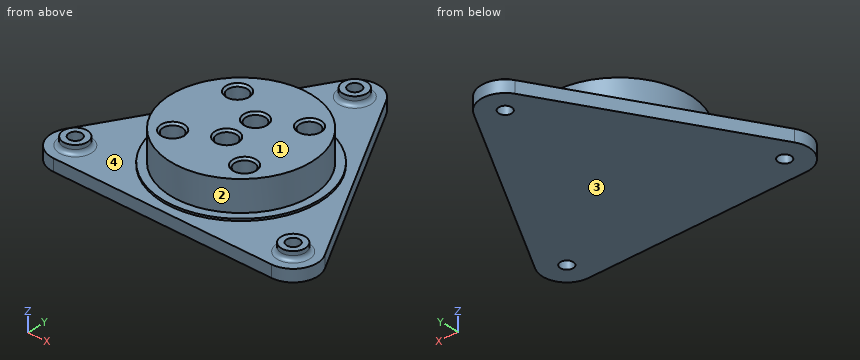
```python
from build123d import *

# Parameters (mm, degrees)
SKETCH2_R           = 1.6
CUT_EXTRUDE1_DEPTH  = 65.58327957
SKETCH3_R           = 2.4
CUT_EXTRUDE2_DEPTH  = 4
SKETCH5_OUTSIDE_W   = 117.55
SKETCH5_OUTSIDE_H   = 117.55
CUT_EXTRUDE4_DEPTH  = 65.140470843
CHAMFER1_SIZE       = 0.5
SKETCH6_R           = 3
SKETCH6_R_2         = 1.6
BOSS_EXTRUDE1_DEPTH = 2
FILLET1_R           = 1
SKETCH7_R           = 1.75
CUT_EXTRUDE5_DEPTH  = 6


with BuildPart() as part:
    # Sketch1 → Revolve1 (revolve)
    with BuildSketch(Plane(origin=(0, 0, 0), x_dir=(0, 0, -1), z_dir=(1, 0, 0)), mode=Mode.PRIVATE) as revolve1_sk:
        Polygon((0, 0), (0, 45), (-3, 45), (-3, 19.5), (-3.5, 19.5), (-3.5, 17.5), (-11, 17.5), (-11, 0), align=None)
    revolve(revolve1_sk.sketch.rotate(Axis((0, 0, 11), (0, 0, -1)), 90), axis=Axis((0, 0, 11), (0, 0, -1)))

    # Sketch2 → Cut-Extrude1 (cut, through all)
    with BuildSketch(Plane(origin=(0, 0, 0), x_dir=(-1, 0, 0), z_dir=(0, 0, -1))):
        with Locations(Location((0, 31.5, 0), (0, 0, 90))):
            Circle(SKETCH2_R)
        with Locations(Location((27.279800219, -15.75, 0), (0, 0, 90))):
            Circle(SKETCH2_R)
        with Locations(Location((-27.279800219, -15.75, 0), (0, 0, 90))):
            Circle(SKETCH2_R)
    extrude(amount=-CUT_EXTRUDE1_DEPTH, mode=Mode.SUBTRACT)

    # Sketch3 → Cut-Extrude2 (cut)
    with BuildSketch(Plane.XY.offset(11)):
        with Locations((0, 4)):
            Circle(SKETCH3_R)
        with Locations((0, -4)):
            Circle(SKETCH3_R)
        with Locations((-9, 9)):
            Circle(SKETCH3_R)
        with Locations((9, 9)):
            Circle(SKETCH3_R)
        with Locations((9, -9)):
            Circle(SKETCH3_R)
        with Locations((-9, -9)):
            Circle(SKETCH3_R)
    extrude(amount=-CUT_EXTRUDE2_DEPTH, mode=Mode.SUBTRACT)

    # Sketch5 outside → Cut-Extrude4 (cut, through all)
    with BuildSketch(Plane(origin=(0, 0, 3), x_dir=(-1, 0, 0), z_dir=(0, 0, -1))):
        Rectangle(SKETCH5_OUTSIDE_W, SKETCH5_OUTSIDE_H)
        with BuildLine():
            Line((-5.196152423, 34.5), (-32.475952642, -12.75))
            ThreePointArc((-32.475952642, -12.75), (-32.475952642, -18.75), (-27.279800219, -21.75))
            Line((-27.279800219, -21.75), (27.279800219, -21.75))
            ThreePointArc((27.279800219, -21.75), (32.475952642, -18.75), (32.475952642, -12.75))
            Line((32.475952642, -12.75), (5.196152423, 34.5))
            ThreePointArc((5.196152423, 34.5), (0, 37.5), (-5.196152423, 34.5))
        make_face(mode=Mode.SUBTRACT)
    extrude(amount=CUT_EXTRUDE4_DEPTH, mode=Mode.SUBTRACT)

    # Chamfer1
    chamfer1_edges = [part.edges().sort_by_distance(p)[0] for p in [
        (-2.4, -4, 11),
        (-11.4, 9, 11),
        (6.6, 9, 11),
        (6.6, -9, 11),
        (-11.4, -9, 11),
        (-2.4, 4, 11),
    ]]
    chamfer(chamfer1_edges, length=CHAMFER1_SIZE)

    # Sketch6 → Boss-Extrude1 (add)
    # profile 1 of 3: a face of its own
    with BuildSketch(Plane.XY.offset(3)):
        with Locations(Location((0, 31.5, 0), (0, 0, 180))):
            Circle(SKETCH6_R)
        with Locations(Location((0, 31.5, 0), (0, 0, 90))):
            Circle(SKETCH6_R_2, mode=Mode.SUBTRACT)
    # profile 2 of 3: a face of its own
    with BuildSketch(Plane.XY.offset(3)):
        with Locations(Location((-27.279800219, -15.75, 0), (0, 0, 180))):
            Circle(SKETCH6_R)
        with Locations(Location((-27.279800219, -15.75, 0), (0, 0, 90))):
            Circle(SKETCH6_R_2, mode=Mode.SUBTRACT)
    # profile 3 of 3: a face of its own
    with BuildSketch(Plane.XY.offset(3)):
        with Locations(Location((27.279800219, -15.75, 0), (0, 0, 180))):
            Circle(SKETCH6_R)
        with Locations(Location((27.279800219, -15.75, 0), (0, 0, 90))):
            Circle(SKETCH6_R_2, mode=Mode.SUBTRACT)
    extrude(amount=BOSS_EXTRUDE1_DEPTH)

    # Fillet1
    fillet1_edges = [part.edges().sort_by_distance(p)[0] for p in [
        (30.279800219, -15.75, 3),
        (-24.279800219, -15.75, 3),
        (3, 31.5, 3),
    ]]
    fillet(fillet1_edges, radius=FILLET1_R)

    # Sketch7 → Cut-Extrude5 (cut)
    with BuildSketch(Plane.XY.offset(11)):
        with Locations((-9, 9)):
            Circle(SKETCH7_R)
        with Locations((0, 4)):
            Circle(SKETCH7_R)
        with Locations((9, 9)):
            Circle(SKETCH7_R)
        with Locations((9, -9)):
            Circle(SKETCH7_R)
        with Locations((-9, -9)):
            Circle(SKETCH7_R)
        with Locations((0, -4)):
            Circle(SKETCH7_R)
    extrude(amount=-CUT_EXTRUDE5_DEPTH, mode=Mode.SUBTRACT)


solid = part.part
```
Model file for the job. Use its own axes, mm. Face numbers are marked on the shaded views. A direction names the side the tool comes from. Coordinates: 2 decimals unless noted, no trailing zeros. Order: outer loops, then holes, each group sorted by start corner. A loop starts at its lowest first (then second) coordinate and runs counter-clockwise, first axis right, second up. Notation, with made-up numbers: M 1.5,62.5 L 48.5,62.5 A17 ccw 48.5,85.5 Z; hole C -3,56 d10. An arc over 180 degrees is marked long. Answer as CSV lines item,"result".
(1) Flat gauge pins, fed straight in: pin 1 (2 mm diameter, centred on x = -20, z = 2, fed in from +Y); pin 2 (1.8 mm diameter, centred on x = -0.5, y = 5, fed in from +Z); pin 3 (4 mm diameter, centred on y = 10, z = 4.5, fed in from -X) (3 decimals); pin 4 (2.5 mm diameter, centred on x = 27.28, y = -15.75, fed in from -Z). Where does each tip first touch, or does it go through?
Geometry says:
pin 1,"stops at y = 10.59"
pin 2,"stops at z = 7"
pin 3,"stops at x = -20.105"
pin 4,"passes through"
(2) Band-saw the part on C-C, the plane y = -15.75. State how many separate pieces and enclosed holes the cut face has, then the cut area to 3 significant figures.
Geometry says:
separate pieces,"3"
enclosed holes,"0"
area,"318 mm2"
(3) Pull direction X, two halves, no side cores. Call the marked faces 3 and 4: +X half, -X half, draft (parallel to the pull), parting line (faces both ways), or undercut.
Geometry says:
face 3,"draft"
face 4,"undercut"
(4) Band-saw the part on A-A, the plane z = 9.75. List the corners of the cut face in (x, y), then the cut area to 3 significant figures.
Geometry says:
outline,"C 0,0 d35; hole C -9,-9 d4.8; hole C -9,9 d4.8; hole C 0,-4 d4.8; hole C 0,4 d4.8; hole C 9,-9 d4.8; hole C 9,9 d4.8"
area,"854 mm2"
(5) Wall check: line 1 along X through (y, z) = (-15.75, 1.1); line 2 along Y through (x, z) = (9, 7.9); line 3 along X through (y, z) = (-15.75, 4.55). Give the ranges that are in metal, low to high.
Geometry says:
line 1,"x = -33.28 to -28.88, -25.68 to 25.68, 28.88 to 33.28"
line 2,"y = -15.01 to -11.4, -6.6 to 6.6, 11.4 to 15.01"
line 3,"x = -30.28 to -28.88, -25.68 to -24.28, -7.63 to 7.63, 24.28 to 25.68, 28.88 to 30.28"
(6) Band-saw the part on B-B, the plane y = 31.5. List the corners of the cut face in (x, z).
Geometry says:
outline,"M -6.93,0 L -1.6,0 L -1.6,5 L -3,5 L -3,4 A1 cw -4,3 L -6.93,3 Z; M 1.6,0 L 6.93,0 L 6.93,3 L 4,3 A1 cw 3,4 L 3,5 L 1.6,5 Z"
(7) 3-axis set-ups, long thin cutter, end or side, ignore diameter. For the marked faces 1 and 2: which of +Z, -Z, +X, -X, +Y, -Y reach the whole face in a straight line?
Geometry says:
face 1,"+Z, +X, -X, +Y, -Y"
face 2,"+Z"
